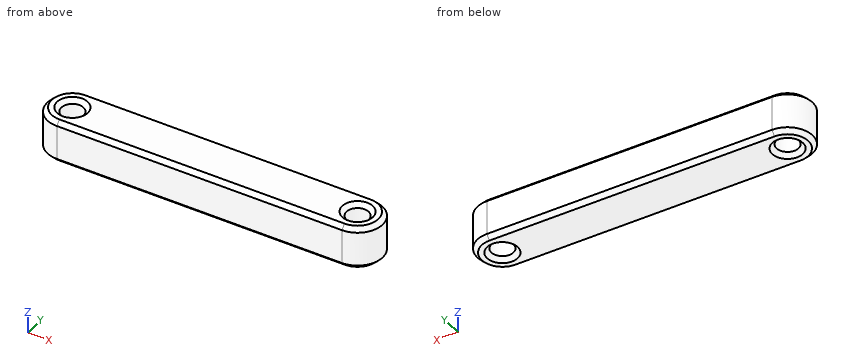
```python
from build123d import *

# Parameters (mm, degrees)
SKETCH_1_R      = 1.55
EXTRUDE_1_DEPTH = 6
CHAMFER_1_SIZE  = 0.6


with BuildPart() as part:
    # 草图1 → 凸台-拉伸1 (new body)
    with BuildSketch(Plane.XY):
        with BuildLine():
            ThreePointArc((0, 3.5), (-3.5, 0), (0, -3.5))
            Line((0, -3.5), (40, -3.5))
            ThreePointArc((40, -3.5), (43.5, 0), (40, 3.5))
            Line((40, 3.5), (0, 3.5))
        make_face()
        Circle(SKETCH_1_R, mode=Mode.SUBTRACT)
        with Locations((40, 0)):
            Circle(SKETCH_1_R, mode=Mode.SUBTRACT)
    extrude(amount=EXTRUDE_1_DEPTH)

    # 倒角1
    chamfer_1_edges = [part.edges().sort_by_distance(p)[0] for p in [
        (43.5, 0, 6),
        (20, 3.5, 6),
        (-3.5, 0, 6),
        (38.45, 0, 6),
        (-1.55, 0, 6),
        (20, -3.5, 6),
        (-1.55, 0, 0),
        (38.45, 0, 0),
        (-3.5, 0, 0),
        (20, 3.5, 0),
        (43.5, 0, 0),
        (20, -3.5, 0),
    ]]
    chamfer(chamfer_1_edges, length=CHAMFER_1_SIZE)


solid = part.part
```
Model file for the job. Use its own axes, mm. Coordinates: 2 decimals unless noted, no trailing zeros. Order: outer loops, then holes, each group sorted by start corner. A loop starts at its lowest first (then second) coordinate and runs counter-clockwise, first axis right, second up. Notation, with made-up numbers: (75, 45.5) - (131, 45.5) arc R23 cw to (131, 80.5) - close; hole circle Ø8 at (80, -5). An arc over 180 degrees is marked (long way). Return JSON: item names as keys, results as strings. Group by question number.
1) Flat gauge pins, fed straight in: P1, Ø3, axis at y = 2, z = 5, coming from the +X side; P2, Ø1.5, axis at y = -1.5, z = 4, coming from the -X side. Where does each tip first touch, or does it go through?
2) Saw through at A-A, the plane y = 0. Write the cut outline in (x, z), plus the area to 3 significant figures.
3) Saw through at B-B, the plane z = 1.25. Write the cut outline in (x, y), plus the area to 3 significant figures.
4) Saw through at C-C, the plane x = 20.5. Write the cut outline in (y, z).
5) Probe line 1 (Y direction, x = 40, z = 4.1); line 2 (X direction, y = 1, z = 3.1); line 3 (X direction, y = -1.25, z = 5). List the from-to ranges inside material, lowest first. Write a range as from..to.
Values found:
{
 "1": {"P1": "stops at x = 43.46", "P2": "stops at x = -3.42"},
 "2": {"outline": "(-3.5, 0.6) - (-2.9, 0) - (-2.15, 0) - (-1.55, 0.6) - (-1.55, 5.4) - (-2.15, 6) - (-2.9, 6) - (-3.5, 5.4) - close; (1.55, 0.6) - (2.15, 0) - (37.85, 0) - (38.45, 0.6) - (38.45, 5.4) - (37.85, 6) - (2.15, 6) - (1.55, 5.4) - close; (41.55, 0.6) - (42.15, 0) - (42.9, 0) - (43.5, 0.6) - (43.5, 5.4) - (42.9, 6) - (42.15, 6) - (41.55, 5.4) - close", "area": "243 mm²"},
 "3": {"outline": "(0, -3.5) - (40, -3.5) arc R3.5 ccw to (40, 3.5) - (0, 3.5) arc R3.5 ccw to start; hole circle Ø3.1 at (0, 0); hole circle Ø3.1 at (40, 0)", "area": "303 mm²"},
 "4": {"outline": "(-3.5, 0.6) - (-2.9, 0) - (2.9, 0) - (3.5, 0.6) - (3.5, 5.4) - (2.9, 6) - (-2.9, 6) - (-3.5, 5.4) - close"},
 "5": {"line 1": "y = -3.5..-1.55, 1.55..3.5", "line 2": "x = -3.35..-1.18, 1.18..38.82, 41.18..43.35", "line 3": "x = -3.27..-0.92, 0.92..39.08, 40.92..43.27"}
}
